The listing builds one solid part. Answer for the finished solid, in the listing's coordinates (mm). A direction names the side the tool comes from. Give positions to 0.01 mm unless a question says otherwise; leave off trailing zeros. Loops run counter-clockwise (first coordinate to the right, second up) from the corner with the lowest first, then second, coordinate; pieces in that order, holes last.
Item 1: Section A-A, the plane y = 0 is taken. Give the vertices of the cut face in (x, z).
Item 2: The mould has two halves that part along Y. Classify faces 1 (the face through (4.04, 5.954, 1.875)), 2 (the face through (2.5, 0, 0)), 3 (the face through (15, 0, 0)): pulls with the +Y half, pulls with the -Y half, needs draft (parallel to the pull), parting line crosses it, or undercut.
Item 3: Section C-C, the plane x = 11.75 is taken. Give the vertices of the cut face in (y, z).
Item 4: Each of these flat-tipped pins is pushed along its axis until it touches: pin 1 Ø2 at (x, y) = (8.5, 4.5) entering from -Z; pin 2 Ø1 at (x, y) = (5.5, 5) entering from +Z; pin 3 Ø1.5 at (y, z) = (-0.5, 0) entering from -X. Where does it stop, or does it pass through?
Item 5: Section B-B, the plane x = 14 is taken. Give the vertices of the cut face in (y, z).
Item 6: Consider line 1 along Z through (x, y) = (1.35, 0); line 2 along Z through (x, y) = (1.5, 0); line 3 along X through (y, z) = (0.25, -1.25). Determine where each line is inside the solid, lowest interval first.
Item 7: A tool of negligible diameter and unlimited length cuts with its end or side. For faces 4 (the face through (0, 0, -2)), 5 (the face through (1.23, 1.5, 0.07)), from which of +Z, -Z, +X, -X, +Y, -Y can it reach the whole face along a straight path? Write none if from no direction.
from build123d import *

# Parameters (mm, degrees)
F0_R     = 5
F1_DEPTH = 15
F1_TAPER = -17.1
F2_R     = 2
F3_R     = 1
F4_R     = 1.5
F5_DEPTH = 2.5


with BuildPart() as f1:
    # F0 (on Right) → F1 (new body)
    with BuildSketch(Plane.YZ):
        Circle(F0_R)
    extrude(amount=F1_DEPTH, taper=F1_TAPER)

    # F2
    f2_edges = [f1.edges().sort_by_distance(p)[0] for p in [
        (15, -9.614603, 0),
    ]]
    fillet(f2_edges, radius=F2_R)

    # F3
    f3_edges = [f1.edges().sort_by_distance(p)[0] for p in [
        (0, -5, 0),
    ]]
    fillet(f3_edges, radius=F3_R)

    # F4 (on face) → F5 (cut)
    with BuildSketch(Plane(origin=(0, 0, 0), x_dir=(0, -1, 0), z_dir=(-1, 0, 0))):
        Circle(F4_R)
    extrude(amount=-F5_DEPTH, mode=Mode.SUBTRACT)


solid = f1.part
Worked answers:
1. outline: (0, -4.26) arc R1 ccw to (0.71, -5.22) - (12.41, -8.82) arc R2 ccw to (15, -6.91) - (15, 6.91) arc R2 ccw to (12.41, 8.82) - (0.71, 5.22) arc R1 ccw to (0, 4.26) - (0, 1.5) - (2.5, 1.5) - (2.5, -1.5) - (0, -1.5) - close
2. face 1: parting line crosses it
2. face 2: undercut
2. face 3: needs draft
3. outline: circle Ø17.23 at (0, 0)
4. pin 1: stops at z = -6.87
4. pin 2: stops at z = 5
4. pin 3: stops at x = 2.5
5. outline: circle Ø17.28 at (0, 0)
6. line 1: z = -5.42 to -1.5, 1.5 to 5.42
6. line 2: z = -5.46 to -1.5, 1.5 to 5.46
6. line 3: x = 2.5 to 15
7. face 4: +Z, -Z, -X, +Y, -Y
7. face 5: -X
